Part model, mm, in its own coordinate system. A direction names the side the tool comes from. Give positions to 0.01 mm unless a question says otherwise; leave off trailing zeros. Write each loop counter-clockwise with the first axis right and the second up, starting at its lowest first coordinate (ties: lowest second). Pieces come first, ordered by that corner, then holes. Notation, with made-up numbers: (-14, 27) - (4, 27) arc R26 cw to (4, 51) - close; hole circle Ø8 at (78, -8). An arc over 180 degrees is marked (long way). Answer in a Markdown table with one row per item. Add a question column.
1. Which spindle directions (+Z, -Z, +X, -X, +Y, -Y) get a long thin tool onto all of the face, cutting with end or side? Do faces 4 (the flat face through (23, 4, -45.5)), 5 (the cylindrical face through (78, 5, -79)). Say none if no direction does.
2. Pull direction X, two halves, no side cores. Call faces 1 (the cylindrical face through (2, 5, -1)), 2 (the flat face through (80, 5, -40)), 3 (the flat face through (40, 4, -40)): released by +X, released by -X, zero draft, split by the parting line, or undercut.
3. Probe line 1 along Z through (x, y) = (31, 3.5); line 2 along Z through (x, y) = (48, 1.75); line 3 along X through (y, z) = (1, -35). List the from-to ranges inside material, lowest first.
4. Band-saw the part on D-D on y = 2. Write the cut outline in (x, z).
5. Band-saw the part on A-A on x = 34.5. Write the cut outline in (y, z).
6. Band-saw the part on B-B on y = 7. Write the cut outline in (x, z), plus the area to 3 significant figures.
```python
from build123d import *

# Parameters (mm, degrees)
ESQUISSE1_W             = 80
ESQUISSE1_H             = 80
EXTRUSION1_DEPTH        = 10
ESQUISSE2_W             = 24.5
ESQUISSE2_H             = 11
ENL_V_MAT_EXTRU_1_DEPTH = 8
CHANFREIN1_SIZE         = 8
CHANFREIN2_SIZE         = 8
CONG_1_R                = 5
ESQUISSE3_W             = 5
ESQUISSE3_H             = 5
ENL_V_MAT_EXTRU_2_DEPTH = 5


with BuildPart() as part:
    # Esquisse1 → Extrusion1 (new body)
    with BuildSketch(Plane(origin=(0, 0, 0), x_dir=(1, 0, 0), z_dir=(0, 1, 0))):
        with Locations((40, 40)):
            Rectangle(ESQUISSE1_W, ESQUISSE1_H)
    extrude(amount=EXTRUSION1_DEPTH)

    # Esquisse2 → Enlèv. mat.-Extru.1 (cut)
    with BuildSketch(Plane.XZ):
        with Locations((23.75, -40)):
            Rectangle(ESQUISSE2_W, ESQUISSE2_H)
    extrude(amount=-ENL_V_MAT_EXTRU_1_DEPTH, mode=Mode.SUBTRACT)

    # Chanfrein1
    chanfrein1_edges = [part.edges().sort_by_distance(p)[0] for p in [
        (11.5, 0, -40),
    ]]
    chamfer(chanfrein1_edges, length=CHANFREIN1_SIZE - 0.0001)  # a hair under: the kernel refuses the full size

    # Chanfrein2
    chanfrein2_edges = [part.edges().sort_by_distance(p)[0] for p in [
        (36, 0, -40),
    ]]
    chamfer(chanfrein2_edges, length=CHANFREIN2_SIZE - 0.0001)  # a hair under: the kernel refuses the full size

    # Congé1
    cong_1_edges = [part.edges().sort_by_distance(p)[0] for p in [
        (0, 5, -80),
        (80, 5, -80),
        (80, 5, 0),
        (0, 5, 0),
    ]]
    fillet(cong_1_edges, radius=CONG_1_R)

    # Esquisse3 → Enlèv. mat.-Extru.2 (cut)
    with BuildSketch(Plane.XZ):
        with Locations((46.5, -40)):
            Rectangle(ESQUISSE3_W, ESQUISSE3_H)
    extrude(amount=-ENL_V_MAT_EXTRU_2_DEPTH, mode=Mode.SUBTRACT)


solid = part.part
```
Values:
| question | item | result |
|---|---|---|
| 1 | face 4 | -Y |
| 1 | face 5 | -Z, +X, +Y, -Y |
| 2 | face 1 | released by -X |
| 2 | face 2 | released by +X |
| 2 | face 3 | undercut |
| 3 | line 1 | z = -80 to -45.5, -34.5 to 0 |
| 3 | line 2 | z = -80 to -42.5, -37.5 to 0 |
| 3 | line 3 | x = 0 to 4.5, 43 to 80 |
| 4 | outline | (0, -75) arc R5 ccw to (5, -80) - (75, -80) arc R5 ccw to (80, -75) - (80, -5) arc R5 ccw to (75, 0) - (5, 0) arc R5 ccw to (0, -5) - close; hole (5.5, -45.5) - (42, -45.5) - (42, -34.5) - (5.5, -34.5) - close; hole (44, -42.5) - (49, -42.5) - (49, -37.5) - (44, -37.5) - close |
| 5 | outline | (0, -80) - (10, -80) - (10, 0) - (0, 0) - (0, -34.5) - (8, -34.5) - (8, -45.5) - (0, -45.5) - close |
| 6 | outline | (0, -75) arc R5 ccw to (5, -80) - (75, -80) arc R5 ccw to (80, -75) - (80, -5) arc R5 ccw to (75, 0) - (5, 0) arc R5 ccw to (0, -5) - close; hole (10.5, -45.5) - (37, -45.5) - (37, -34.5) - (10.5, -34.5) - close |
| 6 | area | 6,090 mm² |
